from build123d import *

# Parameters (mm, degrees)
F0_R     = 3.81
F0_R_2   = 1.27
F1_DEPTH = 19.05
F2_DEPTH = 6.35
F3_DEPTH = 5.08


with BuildPart() as f1:
    # F0 (on Front) → F1 (new body)
    with BuildSketch(Plane.XZ):
        Circle(F0_R)
        Circle(F0_R_2, mode=Mode.SUBTRACT)
    extrude(amount=F1_DEPTH)

    # F2 (add): a face of the model
    f2_faces = [f1.faces().sort_by_distance(p)[0] for p in [
        (-3.7022369265, -19.05, 0),
    ]]
    extrude(f2_faces, amount=F2_DEPTH)

    # F3 (cut): a face of the model
    f3_faces = [f1.faces().sort_by_distance(p)[0] for p in [
        (-3.7022369265, -25.4, 0),
    ]]
    extrude(f3_faces, amount=-F3_DEPTH, mode=Mode.SUBTRACT)


solid = f1.part
Design review of the part built by this model. Coordinates are the model's own, in mm. Coordinates: 2 decimals unless noted, no trailing zeros. Loops run counter-clockwise (first coordinate to the right, second up) from the corner with the lowest first, then second, coordinate; pieces in that order, holes last.
Item 1: Clearance check with flat-ended pins moving along their axes: pin 1 (2 mm diameter, centred on x = -1.5, y = -6.5, fed in from +Z); pin 2 (1.5 mm diameter, centred on x = -3, y = -4, fed in from +Z); pin 3 (1.5 mm diameter, centred on y = -7.5, z = -1.5, fed in from +X); pin 4 (2 mm diameter, centred on x = 0, z = 0, fed in from +Y). State where each tip first meets the part, or that it passes through.
Completed:
pin 1: stops at z = 3.78
pin 2: stops at z = 3.07
pin 3: stops at x = 3.74
pin 4: passes through
Item 2: Draft analysis for pull direction X (two halves, no side actions). For faces 1 (the cylindrical face through (-0.83, -10.02, -3.72)), 2 (the cylindrical face through (-0.17, -10.02, 1.26)), 3 (the flat face through (2, 0, 0)), state which applies: pulls with the +X half, pulls with the -X half, needs draft (parallel to the pull), parting line crosses it, or undercut.
Completed:
face 1: parting line crosses it
face 2: undercut
face 3: needs draft
Item 3: Add section D-D (z = 2.5). Write out the cut boundary in (x, y).
Completed:
outline: (-2.88, -20.32) - (2.88, -20.32) - (2.88, 0) - (-2.88, 0) - close
Item 4: Wall thickness on L1, parallel to Z at x = 0, y = -16; L2, parallel to X at y = -15.5, z = 0.25; L3, parallel to X at y = -16, z = -0.75: over which ranges is each line inside the solid? List them lowest first.
Completed:
L1: z = -3.81 to -1.27, 1.27 to 3.81
L2: x = -3.8 to -1.25, 1.25 to 3.8
L3: x = -3.74 to -1.02, 1.02 to 3.74
Item 5: Add section A-A (z = 0). Write out the cut boundary in (x, y), and give its area (3 significant figures).
Completed:
outline: (-3.81, -20.32) - (-1.27, -20.32) - (-1.27, 0) - (-3.81, 0) - close; (1.27, -20.32) - (3.81, -20.32) - (3.81, 0) - (1.27, 0) - close
area: 103 mm2
Item 6: Add section C-C (y = -11). Write out the cut boundary in (x, z).
Completed:
outline: circle Ø7.62 at (0, 0); hole circle Ø2.54 at (0, 0)
Item 7: Add section B-B (x = 0). Write out the cut boundary in (y, z).
Completed:
outline: (-20.32, -3.81) - (0, -3.81) - (0, -1.27) - (-20.32, -1.27) - close; (-20.32, 1.27) - (0, 1.27) - (0, 3.81) - (-20.32, 3.81) - close
